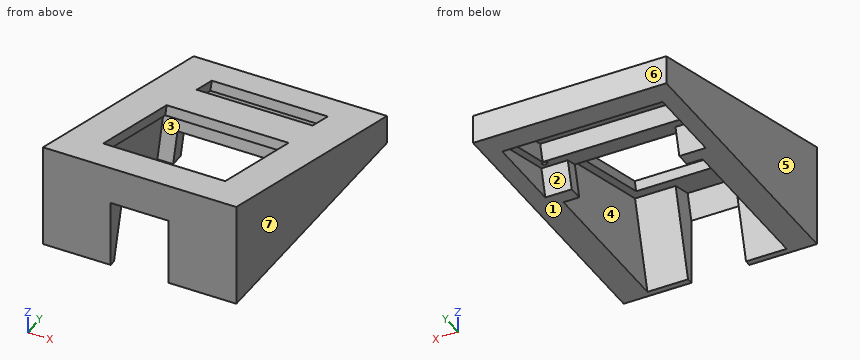
from build123d import *

# Parameters (mm, degrees)
BOSS_EXTRUDE1_DEPTH = 50
SKETCH5_W           = 15
SKETCH5_H           = 144.888873943
BOSS_EXTRUDE2_DEPTH = 50
SKETCH3_W           = 63.082028678
SKETCH3_H           = 63.082028678
SKETCH3_W_2         = 60
SKETCH3_H_2         = 15
CUT_EXTRUDE1_DEPTH  = 153.964709483
CUT_EXTRUDE2_START  = -5
SKETCH4_W           = 75
SKETCH4_H           = 27
CUT_EXTRUDE2_DEPTH  = 148.964709483
CUT_EXTRUDE3_START  = -14
SKETCH6_W           = 83
SKETCH6_H           = 40
CUT_EXTRUDE3_DEPTH  = 100
SKETCH7_R           = 1.5
CUT_EXTRUDE4_DEPTH  = 10
SKETCH8_W           = 55.690082514
SKETCH8_H           = 14
CUT_EXTRUDE5_DEPTH  = 153.277751166


with BuildPart() as part:
    # Sketch1 → Boss-Extrude1 (new, symmetric)
    with BuildSketch(Plane(origin=(0, 0, 0), x_dir=(0, 0, -1), z_dir=(1, 0, 0))):
        Polygon((0, 0), (0, 144.888873943), (-38.822856765, 0), align=None)
    extrude(amount=BOSS_EXTRUDE1_DEPTH, both=True)

    # Sketch5 → Boss-Extrude2 (add, symmetric)
    with BuildSketch(Plane(origin=(0, 0, 0), x_dir=(0, 0, -1), z_dir=(1, 0, 0))):
        with Locations((7.5, 72.444436972)):
            Rectangle(SKETCH5_W, SKETCH5_H)
    extrude(amount=BOSS_EXTRUDE2_DEPTH, both=True)

    # Sketch3 → Cut-Extrude1 (cut, through all)
    with BuildSketch(Plane(origin=(0, 9.705714191, 36.222218486), x_dir=(1, 0, 0), z_dir=(0, 0.25881904510251436, 0.96592582628907))):
        with Locations((0, 45.951905284)):
            Rectangle(SKETCH3_W, SKETCH3_H)
        with Locations((0, 111.951905284)):
            Rectangle(SKETCH3_W_2, SKETCH3_H_2)
    extrude(amount=-CUT_EXTRUDE1_DEPTH, mode=Mode.SUBTRACT)

    # Sketch4 → Cut-Extrude2 (cut, through all)
    with BuildSketch(Plane(origin=(0, 9.705714191, 36.222218486), x_dir=(1, 0, 0), z_dir=(0, 0.25881904510251436, 0.96592582628907)).offset(CUT_EXTRUDE2_START)):
        Polygon((-36, 84.951905284), (36, 84.951905284), (36, 6.951905284), (15, 6.951905284), (15, -5.048094716), (-15, -5.048094716), (-15, 6.951905284), (-36, 6.951905284), align=None)
        with Locations((0, 111.951905284)):
            Rectangle(SKETCH4_W, SKETCH4_H)
    extrude(amount=-CUT_EXTRUDE2_DEPTH, mode=Mode.SUBTRACT)

    # Sketch6 → Cut-Extrude3 (cut)
    with BuildSketch(Plane(origin=(0, 9.705714191, 36.222218486), x_dir=(1, 0, 0), z_dir=(0, 0.25881904510251436, 0.96592582628907)).offset(CUT_EXTRUDE3_START)):
        with Locations((0, 111.951905284)):
            Rectangle(SKETCH6_W, SKETCH6_H)
    extrude(amount=-CUT_EXTRUDE3_DEPTH, mode=Mode.SUBTRACT)

    # Sketch7 → Cut-Extrude4 (cut)
    with BuildSketch(Plane(origin=(0, 6.08224756, 22.699256918), x_dir=(-1, 0, 0), z_dir=(0, -0.25881904510251436, -0.96592582628907))):
        with Locations(Location((37.5, 127.451905284, 0), (0, 0, 90))):
            Circle(SKETCH7_R)
        with Locations(Location((-37.5, 127.451905284, 0), (0, 0, 270))):
            Circle(SKETCH7_R)
        with Locations(Location((37.5, 96.451905284, 0), (0, 0, 270))):
            Circle(SKETCH7_R)
        with Locations(Location((-37.5, 96.451905284, 0), (0, 0, 90))):
            Circle(SKETCH7_R)
    extrude(amount=-CUT_EXTRUDE4_DEPTH, mode=Mode.SUBTRACT)

    # Sketch8 → Cut-Extrude5 (cut, through all)
    with BuildSketch(Plane(origin=(0, 6.08224756, 22.699256918), x_dir=(-1, 0, 0), z_dir=(0, -0.25881904510251436, -0.96592582628907))):
        with Locations((0, 91.951905284)):
            Rectangle(SKETCH8_W, SKETCH8_H)
    extrude(amount=CUT_EXTRUDE5_DEPTH, mode=Mode.SUBTRACT)


solid = part.part
For this review, take the finished solid that the model builds, in its own axes (mm). Face numbers are marked on the shaded views. A direction names the side the tool comes from. Give positions to 0.01 mm unless a question says otherwise; leave off trailing zeros. Loops run counter-clockwise (first coordinate to the right, second up) from the corner with the lowest first, then second, coordinate; pieces in that order, holes last.
Item 1: Take a section at D-D, the plane y = 36.5. State the section outline as (x, z) points, and give its area (3 significant figures).
Item 2: Draft analysis for pull direction X (two halves, no side actions). For the marked faces 4, 5, 6 and 7, state which applies: +X half, -X half, draft (parallel to the pull), parting line (faces both ways), or undercut.
Item 3: Insertion check: pin 1 (6 mm diameter, centred on x = 16, y = 112, fed in from +Z); pin 2 (10 mm diameter, centred on x = 9, y = 95, fed in from -Z); pin 3 (17 mm diameter, centred on y = 62.5, z = 26, fed in from -X); pin 4 (2 mm diameter, centred on x = -27, z = 23.5, fed in from +Y). Each pin has a flat end and moves straight along its axis. Give the tip position at first contact, or say it passes through.
Item 4: For line 1 along X through (y, z) = (16, 23.5); line 2 along Y through (x, z) = (-16.5, -4.5); line 3 along Y through (x, z) = (17.5, -13), list the stretches that pass through material, from the lowest coordinate up.
Item 5: Tool access review of the marked faces 1, 2 and 3: name each direction out of +Z, -Z, +X, -X, +Y, -Y from which nothing blocks a thin tool from reaching the whole face with its end or side.
Item 6: Take a section at A-A, the plane x = 25. State the section outline as (y, z) points, and give its area (3 significant figures).
Item 7: Take a section at C-C, the plane z = 13.5. State the section outline as (x, y) points, and give its area (3 significant figures).
Item 8: Take a section at B-B, the plane y = 81.5. State the section outline as (x, z) points (3 decimals).
Calculated:
1. outline: (-50, -15) - (-36, -15) - (-36, 23.87) - (-31.54, 23.87) - (-31.54, 29.04) - (-50, 29.04) - close; (31.54, 23.87) - (36, 23.87) - (36, -15) - (50, -15) - (50, 29.04) - (31.54, 29.04) - close
1. area: 1,280 mm2
2. face 4: undercut
2. face 5: -X half
2. face 6: draft
2. face 7: +X half
3. pin 1: stops at z = 9.62
3. pin 2: stops at z = -2.47
3. pin 3: stops at x = -50
3. pin 4: stops at y = 13.76
4. line 1: x = -50 to -36, 36 to 50
4. line 2: y = 0 to 5.99, 128.67 to 144.89
4. line 3: y = 0 to 3.71, 133.12 to 144.89
5. face 1: -Z, +X, -X, +Y, -Y
5. face 2: -Z
5. face 3: none
6. outline: (0, -15) - (3.18, -15) - (15.13, 29.59) - (22.33, 27.66) - (23.63, 32.49) - (0, 38.82) - close; (83.26, 11.34) - (90.47, 9.41) - (88.14, 0.71) - (101.18, -2.78) - (103.51, 5.91) - (109.3, 4.36) - (110.6, 9.19) - (84.56, 16.17) - close; (123.79, 0.48) - (129.59, -1.08) - (127.26, -9.77) - (133.54, -11.45) - (132.59, -15) - (144.89, -15) - (144.89, 0) - (125.09, 5.31) - close
6. area: 1,100 mm2
7. outline: (-50, 0) - (-15, 0) - (-15, 10.81) - (-36, 10.81) - (-36, 75.19) - (-31.54, 75.19) - (-31.54, 83.84) - (31.54, 83.84) - (31.54, 75.19) - (36, 75.19) - (36, 10.81) - (15, 10.81) - (15, 0) - (50, 0) - (50, 94.51) - (-50, 94.51) - close
7. area: 3,950 mm2
8. outline: (-50, -15) - (-36, -15) - (-36, 11.809) - (-31.541, 11.809) - (-31.541, 16.985) - (-50, 16.985) - close; (31.541, 11.809) - (36, 11.809) - (36, -15) - (50, -15) - (50, 16.985) - (31.541, 16.985) - close
